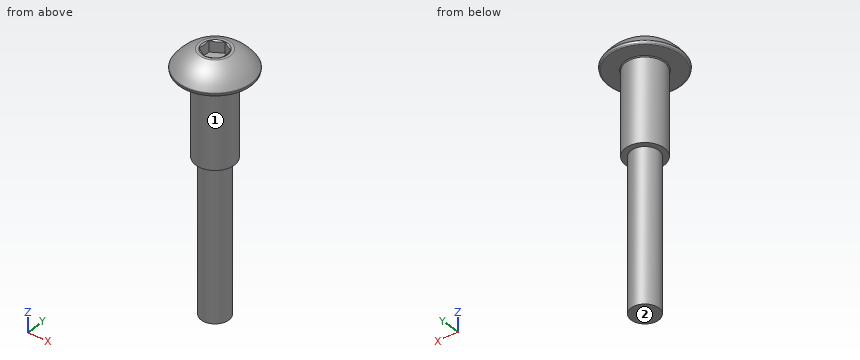
```python
from build123d import *

# Parameters (mm, degrees)
CUT_EXTRUDE1_DEPTH = 1.21539
FILLET1_R          = 0.11049
SKETCH10_R         = 3.811240777
SKETCH10_R_2       = 1.4874875
CUT_EXTRUDE4_DEPTH = 16.4


# Read off the part's stored shape, not the designer's step: Split1
with BuildPart() as part:
    # Sketch3 → Revolve1 (revolve)
    with BuildSketch(Plane(origin=(0, 0, 0), x_dir=(0, 0, -1), z_dir=(1, 0, 0)), mode=Mode.PRIVATE) as revolve1_sk:
        with BuildLine():
            Line((-13.8049, 0), (-13.8049, 1.666875))
            ThreePointArc((-13.8049, 1.666875), (-13.052170588, 2.967189774), (-11.92657, 3.9624))
            Line((-11.92657, 3.9624), (-11.5951, 3.903952896))
            Line((-11.5951, 3.903952896), (-11.5951, 2.0828))
            Line((-11.5951, 2.0828), (13.2095875, 2.0828))
            Line((13.2095875, 2.0828), (13.8049, 1.4874875))
            Line((13.8049, 1.4874875), (13.8049, 0))
            Line((13.8049, 0), (-13.8049, 0))
        make_face()
    revolve(revolve1_sk.sketch.rotate(Axis((0, 0, 13.8049), (0, 0, -1)), 90), axis=Axis((0, 0, 13.8049), (0, 0, -1)))

    # Sketch4 → Cut-Extrude1 (cut)
    with BuildSketch(Plane.XY.offset(13.8049)):
        Polygon((-1.190625, -0.687407664), (0, -1.374815329), (1.190625, -0.687407664), (1.190625, 0.687407664), (0, 1.374815329), (-1.190625, 0.687407664), align=None)
    extrude(amount=-CUT_EXTRUDE1_DEPTH, mode=Mode.SUBTRACT)

    # Cut-Extrude2 cone 1 section (through the dimple's axis) → Cut-Extrude2 (revolve, cut)
    with BuildSketch(Plane(origin=(0, 0, 13.8049), x_dir=(0, -1, 0), z_dir=(1, 0, 0))):
        Polygon((0, 0), (1.374815329, 0), (0, 0.79375), align=None)
    revolve(axis=Axis((0, 0, 13.8049), (0, 0, -1)), mode=Mode.SUBTRACT)

    # Fillet1
    fillet1_edges = [part.edges().sort_by_distance(p)[0] for p in [
        (-3.903952896, 0, 11.5951),
        (-3.9624, 0, 11.92657),
    ]]
    fillet(fillet1_edges, radius=FILLET1_R)


with BuildPart() as body_2:
    # Split1: the piece on the far side of the plane
    add(part.part)
    split(bisect_by=Plane.XY.offset(11.5951), keep=Keep.BOTTOM)


with BuildPart() as part_1:
    add(part.part)

    # Split1
    split(bisect_by=Plane.XY.offset(11.5951), keep=Keep.TOP)

    add(body_2.part)  # Boss-Extrude1 merges body 2
    # Boss-Extrude1 cone 1 section (through the dimple's axis) → Boss-Extrude1 (revolve)
    with BuildSketch(Plane(origin=(0, 0, 11.5951), x_dir=(0, -1, 0), z_dir=(1, 0, 0))):
        Polygon((0, 0), (2.168725958, 0), (0, 2.168725958), align=None)
    revolve(axis=Axis((0, 0, 11.5951), (0, 0, -1)))

    # Sketch10 → Cut-Extrude4 (cut)
    with BuildSketch(Plane(origin=(0, 0, -13.8049), x_dir=(-1, 0, 0), z_dir=(0, 0, -1))):
        Circle(SKETCH10_R)
        Circle(SKETCH10_R_2, mode=Mode.SUBTRACT)
    extrude(amount=-CUT_EXTRUDE4_DEPTH, mode=Mode.SUBTRACT)


solid = part_1.part
```
Geometry: final body of the model. Coordinates: model frame, mm. Face numbers are marked on the shaded views. Round coordinates to 2 decimals unless told otherwise and drop trailing zeros. Loops run counter-clockwise (first coordinate to the right, second up) from the corner with the lowest first, then second, coordinate; pieces in that order, holes last. Notation, with made-up numbers: (-32.5, 8.25) -> (-20.5, 8.25) arc R9 cw to (-20.5, 20.25) -> close; hole circle Ø1 at (17.25, -38). An arc over 180 degrees is marked (long way). Use one line per item in the form item = value.
Item 1: Cut plane B-B on z = 4.5. Output: boundary loops of the cut face in (x, y), then the cut area to 3 significant figures.
Evaluation:
outline = circle Ø4.17 at (0, 0)
area = 13.6 mm2
Item 2: Cut plane A-A on z = -8.75. Output: boundary loops of the cut face in (x, y), then the cut area to 3 significant figures.
Evaluation:
outline = circle Ø2.97 at (0, 0)
area = 6.95 mm2
Item 3: Draft query along Y for the marked faces 1 and 2. Return one class per face: released by +Y, released by -Y, zero draft, split by the parting line, or undercut.
Evaluation:
face_1 = split by the parting line
face_2 = zero draft
Item 4: Material intervals for probe 1 along Z at (x, y) = (0, 1.25); probe 2 along X at (y, z) = (0, -8.5); probe 3 along Z at (x, y) = (1.5, -2.75), sorted ascending.
Evaluation:
probe_1 = -13.8 to 12.59
probe_2 = -1.49 to 1.49
probe_3 = 11.6 to 12.91
Item 5: Contact query for flat-ended pins moving along their axis: pin 1 Ø1 at (y, z) = (1, -8) entering from +X; pin 2 Ø4 at (y, z) = (-0.5, 6) entering from -X; pin 3 Ø0.7 at (x, y) = (0.5, 0) entering from +Z. Output: stop coordinate, or through.
Evaluation:
pin_1 = 1.4
pin_2 = -2.08
pin_3 = 12.59
